Here's how the part is built. I have some questions about the finished solid (model axes, mm). A direction names the side the tool comes from. Coordinates: 2 decimals unless noted, no trailing zeros. Loops run counter-clockwise (first coordinate to the right, second up) from the corner with the lowest first, then second, coordinate; pieces in that order, holes last. Notation, with made-up numbers: M 6.5,25 L 61.5,25 A7 ccw 61.5,30 Z; hole C 41.25,12.5 d11. An arc over 180 degrees is marked long. Use CSV: the item, a comma, the result in double quotes. Start each with the question number.
Q1. If we section it at D-D (y = 8.89): Please give me the cut outline in (x, z).
Q2. If we section it at C-C (z = -11.5): Please give me the cut outline in (x, y) (1 decimal).
Q3. Please list where these lines run through material, in increasing order: probe 1 along Y at (x, z) = (12.25, -13.97); probe 2 along X at (y, z) = (3, 11.5); probe 3 along Z at (x, y) = (-0.75, 4). Write a range as [from, to].
Q4. For pin 1 Ø2 at (x, y) = (3, 0) entering from -Z; pin 2 Ø2.5 at (x, y) = (-6.02, 6.02) entering from -Z; pin 3 Ø5 at (x, y) = (-6.5, 3.5) entering from +Z, each with a flat end and sliding along its axis, tell me the tip position at first contact or that it passes through.
Q5. Which directions (+Z, -Z, +X, -X, +Y, -Y) give clear straight access to the entire face, cutting with the end or side of a thin tool? Please do faces 5 (the cylindrical face through (-2.75, -12.4, 3.93)), 6 (the cylindrical face through (-8.327, -0.05, 12.074)), 7 (the flat face through (-11.809, -1, -14)), 8 (the flat face through (3, 0, -10.16)).
Q6. If we mould it in two halves opening along Y, with no side actions, what happens to faces 1 (the cylindrical face through (-11.81, 3.72, -8.84)), 2 (the cylindrical face through (8.327, 0.05, 12.074)), 3 (the cylindrical face through (-2.24, 0.86, -11.45)), 4 (the flat face through (0, 0, -12.7))? For each: +Y half, -Y half, draft (parallel to the pull), parting line (faces both ways), or undercut.
Q7. If we section it at B-B (z = 20): Please give me the cut outline in (x, y) (1 decimal).
from build123d import *

# Parameters (mm, degrees)
SKETCH2_R           = 12.7
BOSS_EXTRUDE1_DEPTH = 12.7
SKETCH3_R           = 3.175
SKETCH3_R_2         = 1.5875
BOSS_EXTRUDE2_DEPTH = 1.5875
SKETCH4_R           = 1.5875
BOSS_EXTRUDE3_DEPTH = 12.7
CUT_EXTRUDE1_START  = -12.7
CUT_EXTRUDE1_DEPTH  = 12.7
CUT_EXTRUDE2_DEPTH  = 1.27
CIRPATTERN1_COUNT   = 4
SKETCH7_R           = 1.524
CUT_EXTRUDE3_DEPTH  = 5.08
CUT_EXTRUDE4_START  = -7.62
SKETCH8_R           = 12.7
SKETCH8_R_2         = 12.3825
CUT_EXTRUDE4_DEPTH  = 7.62
SKETCH9_R           = 1.27
CUT_EXTRUDE5_DEPTH  = 2.54
SKETCH11_W          = 0.508
SKETCH11_H          = 2.54
BOSS_EXTRUDE4_DEPTH = 2.54
SKETCH12_R          = 0.381
CUT_EXTRUDE6_DEPTH  = 2.54


with BuildPart() as part:
    # Sketch2 → Boss-Extrude1 (new, symmetric)
    with BuildSketch(Plane.XY):
        Circle(SKETCH2_R)
    extrude(amount=BOSS_EXTRUDE1_DEPTH, both=True)

    # Sketch3 → Boss-Extrude2 (add, symmetric)
    with BuildSketch(Plane.XY.offset(12.7)):
        Circle(SKETCH3_R)
        Circle(SKETCH3_R_2, mode=Mode.SUBTRACT)
    extrude(amount=BOSS_EXTRUDE2_DEPTH, both=True)

    # Sketch4 → Boss-Extrude3 (add)
    with BuildSketch(Plane.XY.offset(12.7)):
        Circle(SKETCH4_R)
    extrude(amount=BOSS_EXTRUDE3_DEPTH)

    # Sketch5 → Cut-Extrude1 (cut)
    with BuildSketch(Plane.XY.offset(25.4).offset(CUT_EXTRUDE1_START)):
        with BuildLine():
            Line((-1.315232014, 0.889), (1.315232014, 0.889))
            ThreePointArc((1.315232014, 0.889), (0, 1.5875), (-1.315232014, 0.889))
        make_face()
    extrude(amount=CUT_EXTRUDE1_DEPTH, mode=Mode.SUBTRACT)

    # Sketch6 → Cut-Extrude2 (cut)
    with BuildSketch(Plane.XY.offset(12.7)):
        with BuildLine():
            ThreePointArc((-4.082142857, 9.868873978), (-4.793434391, 8.634827903), (-3.571875, 7.902299395))
            ThreePointArc((-3.571875, 7.902299395), (0, 8.326790326), (3.571875, 7.902299395))
            ThreePointArc((3.571875, 7.902299395), (4.793434391, 8.634827903), (4.082142857, 9.868873978))
            ThreePointArc((4.082142857, 9.868873978), (0, 10.425764304), (-4.082142857, 9.868873978))
        make_face()
    cut_extrude2 = extrude(amount=-CUT_EXTRUDE2_DEPTH, mode=Mode.SUBTRACT)

    # CirPattern1: Cut-Extrude2 ×4 about axis
    cirpattern1_axis = Axis((0, 0, 0), (0, 0, 1))
    for i in range(1, CIRPATTERN1_COUNT):
        add(cut_extrude2.rotate(cirpattern1_axis, i * 360 / CIRPATTERN1_COUNT), mode=Mode.SUBTRACT)

    # Sketch7 → Cut-Extrude3 (cut)
    with BuildSketch(Plane.XY.offset(12.7)):
        with Locations((-6.016771601, 6.016771601)):
            Circle(SKETCH7_R)
        with Locations((6.016771601, -6.016771601)):
            Circle(SKETCH7_R)
    extrude(amount=-CUT_EXTRUDE3_DEPTH, mode=Mode.SUBTRACT)

    # Sketch8 → Cut-Extrude4 (cut)
    with BuildSketch(Plane(origin=(0, 0, -12.7), x_dir=(-1, 0, 0), z_dir=(0, 0, -1)).offset(CUT_EXTRUDE4_START)):
        with Locations(Location((0, 0, 0), (0, 0, 180))):
            Circle(SKETCH8_R)
        Circle(SKETCH8_R_2, mode=Mode.SUBTRACT)
    extrude(amount=CUT_EXTRUDE4_DEPTH, mode=Mode.SUBTRACT)

    # Sketch9 → Cut-Extrude5 (cut)
    with BuildSketch(Plane(origin=(0, 0, -12.7), x_dir=(-1, 0, 0), z_dir=(0, 0, -1))):
        with Locations((-3.175, 0)):
            Circle(SKETCH9_R)
        with Locations((3.175, 0)):
            Circle(SKETCH9_R)
    extrude(amount=-CUT_EXTRUDE5_DEPTH, mode=Mode.SUBTRACT)

    # Sketch11 → Boss-Extrude4 (add)
    with BuildSketch(Plane(origin=(0, 0, -12.7), x_dir=(-1, 0, 0), z_dir=(0, 0, -1))):
        with Locations((-12.063199611, 0)):
            Rectangle(SKETCH11_W, SKETCH11_H)
    boss_extrude4 = extrude(amount=BOSS_EXTRUDE4_DEPTH)

    # Sketch12 → Cut-Extrude6 (cut)
    with BuildSketch(Plane(origin=(12.317199611, 0, 0), x_dir=(0, 0, -1), z_dir=(1, 0, 0))):
        with Locations((13.97, 0)):
            Circle(SKETCH12_R)
    cut_extrude6 = extrude(amount=-CUT_EXTRUDE6_DEPTH, mode=Mode.SUBTRACT)

    # Mirror1: Boss-Extrude4, Cut-Extrude6 across plane
    add(boss_extrude4.mirror(Plane(origin=(0, 0, 0), x_dir=(0, 0, 1), z_dir=(1, 0, 0))))
    add(cut_extrude6.mirror(Plane(origin=(0, 0, 0), x_dir=(0, 0, 1), z_dir=(1, 0, 0))), mode=Mode.SUBTRACT)


solid = part.part
Results below:
1,outline,"M -9.07,-5.08 L -8.62,-5.08 L -8.62,-12.7 L 8.62,-12.7 L 8.62,-5.08 L 9.07,-5.08 L 9.07,12.7 L 4.83,12.7 L 4.83,11.43 L -4.83,11.43 L -4.83,12.7 L -9.07,12.7 Z"
2,outline,"C 0,0 d24.8; hole C -3.2,0 d2.5; hole C 3.2,0 d2.5"
3,probe 1,"[-1.27, -0.38], [0.38, 1.27]"
3,probe 2,"[-12.34, -10.13], [-8.03, 8.03], [10.13, 12.34]"
3,probe 3,"[-12.7, 12.7]"
4,pin 1,"z = -10.16"
4,pin 2,"z = -12.7"
4,pin 3,"z = 12.7"
5,face 5,"+Z, -Z"
5,face 6,"+Z"
5,face 7,"-Z, +Y, -Y"
5,face 8,"-Z"
6,face 1,"parting line"
6,face 2,"undercut"
6,face 3,"undercut"
6,face 4,"draft"
7,outline,"M -1.3,0.9 A1.6 ccw long 1.3,0.9 Z"
